Check sheet for the modelled part. Datum: model origin and axes. Units: mm. A direction names the side the tool comes from. Give positions to 0.01 mm unless a question says otherwise; leave off trailing zeros. Order: outer loops, then holes, each group sorted by start corner. A loop starts at its lowest first (then second) coordinate and runs counter-clockwise, first axis right, second up.
```python
from build123d import *

# Parameters (mm, degrees)
F1_DEPTH  = 25
F2_W      = 5
F2_H      = 20
F3_DEPTH  = 1
F4_W      = 76.621622
F4_H      = 63
F5_DEPTH  = 1
F7_DEPTH  = 8
F10_DEPTH = 6
F11_R     = 4
F12_DEPTH = 5
F13_W     = 10
F13_H     = 3
F14_DEPTH = 3
F15_W     = 3
F15_H     = 3
F16_DEPTH = 1
F17_W     = 3
F17_H     = 3
F18_DEPTH = 5


with BuildPart() as f1:
    # F0 (on Front) → F1 (new body)
    with BuildSketch(Plane.XZ):
        with BuildLine():
            Line((-40, -74), (40, -74))
            ThreePointArc((40, -74), (43.535534, -72.535534), (45, -69))
            Line((45, -69), (45, 69))
            ThreePointArc((45, 69), (43.535534, 72.535534), (40, 74))
            Line((40, 74), (-40, 74))
            ThreePointArc((-40, 74), (-43.535534, 72.535534), (-45, 69))
            Line((-45, 69), (-45, -69))
            ThreePointArc((-45, -69), (-43.535534, -72.535534), (-40, -74))
        make_face()
    extrude(amount=-F1_DEPTH)

    # F2 (on face) → F3 (join)
    with BuildSketch(Plane.YZ.offset(45)):
        with Locations((12.5, 0)):
            Rectangle(F2_W, F2_H)
    extrude(amount=F3_DEPTH)

    # F4 (on face) → F5 (cut)
    with BuildSketch(Plane.XZ):
        with Locations((0, 37)):
            Rectangle(F4_W, F4_H)
    extrude(amount=-F5_DEPTH, mode=Mode.SUBTRACT)

    # F6 (on face) → F7 (cut)
    with BuildSketch(Plane(origin=(0, 0, -74), x_dir=(1, 0, 0), z_dir=(0, 0, -1))):
        Polygon((3.45, -11.575), (0, -11.575), (-3.45, -11.575), (-3.45, -12.5), (-1.676761, -13.425), (1.676761, -13.425), (3.45, -12.5), align=None)
    extrude(amount=-F7_DEPTH, mode=Mode.SUBTRACT)

    # F9 (on face) → F10 (cut)
    with BuildSketch(Plane.XY.offset(74)):
        with BuildLine():
            ThreePointArc((21.75, 12.5), (20, 14.25), (18.25, 12.5))
            Line((18.25, 12.5), (21.75, 12.5))
        make_face()
        with BuildLine():
            Line((21.75, 12.5), (18.25, 12.5))
            ThreePointArc((18.25, 12.5), (20, 10.75), (21.75, 12.5))
        make_face()
    extrude(amount=-F10_DEPTH, mode=Mode.SUBTRACT)

    # F11 (on Front) → F12 (join)
    with BuildSketch(Plane.XZ):
        Polygon((-20.187831, -27), (-22.687831, -27), (-25.187831, -27), (-25.187831, -34.5), (-32.687831, -34.5), (-32.687831, -37), (-32.687831, -39.5), (-25.187831, -39.5), (-25.187831, -47), (-22.687831, -47), (-20.187831, -47), (-20.187831, -39.5), (-12.687831, -39.5), (-12.687831, -37), (-12.687831, -34.5), (-20.187831, -34.5), align=None)
        with Locations((32.312169, -37)):
            Circle(F11_R)
        with Locations((22.312169, -47)):
            Circle(F11_R)
        with Locations((12.312169, -37)):
            Circle(F11_R)
        with Locations((22.312169, -27)):
            Circle(F11_R)
    extrude(amount=F12_DEPTH)

    # F13 (on face) → F14 (join)
    with BuildSketch(Plane.XZ):
        with Locations((0, -6.875)):
            Rectangle(F13_W, F13_H)
        with Locations((0, -13.75)):
            Rectangle(F13_W, F13_H)
    extrude(amount=F14_DEPTH)

    # F15 (on face) → F16 (cut)
    with BuildSketch(Plane.XY.offset(74)):
        with Locations((-30, 12.5)):
            Rectangle(F15_W, F15_H)
    extrude(amount=-F16_DEPTH, mode=Mode.SUBTRACT)

    # F17 (on face) → F18 (join)
    with BuildSketch(Plane.XY.offset(74)):
        with Locations((-26.967838, 12.45954)):
            Rectangle(F17_W, F17_H)
    extrude(amount=F18_DEPTH)


solid = f1.part
```
(1) Cross-section at B-B on x = -27. Enter the section's corners in (y, z).
Response values:
outline: (-5, -39.5) - (0, -39.5) - (0, -74) - (25, -74) - (25, 74) - (13.96, 74) - (13.96, 79) - (10.96, 79) - (10.96, 74) - (0, 74) - (0, 68.5) - (1, 68.5) - (1, 5.5) - (0, 5.5) - (0, -34.5) - (-5, -34.5) - close
(2) Cross-section at C-C on y = 22.25. Enter the section's corners in (x, z), then the cut area to 3 significant figures.
Response values:
outline: (-45, -69) arc R5 ccw to (-40, -74) - (40, -74) arc R5 ccw to (45, -69) - (45, 69) arc R5 ccw to (40, 74) - (-40, 74) arc R5 ccw to (-45, 69) - close
area: 13,300 mm2
(3) Cross-section at D-D on z = 3. Enter the section's corners in (x, y).
Response values:
outline: (-45, 0) - (45, 0) - (45, 10) - (46, 10) - (46, 15) - (45, 15) - (45, 25) - (-45, 25) - close
(4) Release check for a two-part mould opening along X. For faces 6 (the face through (0, 11.575, -70)), 7 (the face through (-5, -1, -14)), 8 (the face through (-20.188, -2, -31)), 9 (the face through (5, -1, -14)) record: released by +X, released by -X, zero draft, split by the parting line, or undercut.
Response values:
face 6: undercut
face 7: released by -X
face 8: undercut
face 9: released by +X
(5) Gauge pin test, flat ends, axial feed: pin 1 Ø2 at (y, z) = (1.5, 42) entering from +X; pin 2 Ø0.8 at (x, z) = (-30.5, 73.5) entering from -Y; pin 3 Ø0.9 at (x, z) = (-1, -7) entering from -Y; pin 4 Ø5.5 at (y, z) = (-2.5, -31) entering from -X. Record the tip position at first contact, or that the pin passes through.
Response values:
pin 1: stops at x = 45
pin 2: stops at y = 0
pin 3: stops at y = -3
pin 4: stops at x = -45
(6) Set-up check for faces 1 (the face through (0, -1, -12.25)), 2 (the face through (-29, -2, -34.5)), 3 (the face through (0, -1, -5.375)), 4 (the face through (-27, 13.96, 76)), 5 (the face through (-29, -2, -39.5)): record each of +Z, -Z, +X, -X, +Y, -Y from which the full face is reachable in a straight line by a thin tool's end or side.
Response values:
face 1: +X, -X, -Y
face 2: +Z, -X, -Y
face 3: +Z, +X, -X, -Y
face 4: +Z, +X, -X, +Y
face 5: -Z, -X, -Y
(7) Cross-section at A-A on z = -37. Enter the section's corners in (x, y).
Response values:
outline: (-45, 0) - (-32.69, 0) - (-32.69, -5) - (-12.69, -5) - (-12.69, 0) - (8.31, 0) - (8.31, -5) - (16.31, -5) - (16.31, 0) - (28.31, 0) - (28.31, -5) - (36.31, -5) - (36.31, 0) - (45, 0) - (45, 25) - (-45, 25) - close
(8) Material ranges on L1, parallel to Y at x = 20, z = 70; L2, parallel to X at y = 12.5, z = 69.4; L3, parallel to Z at x = 5.5, y = 19.25, recorded low to high.
Response values:
L1: y = 0 to 10.75, 14.25 to 25
L2: x = -44.98 to 18.25, 21.75 to 44.98
L3: z = -74 to 74
